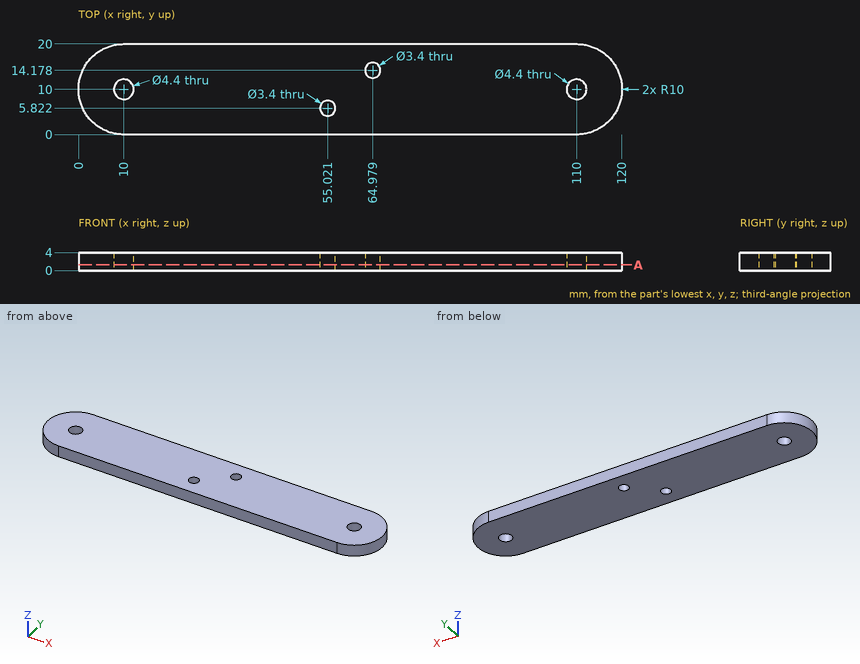
The figure shows three views and two pictorial views of one solid part (mm, origin at its lowest corner). Answer the questions. Give positions to 0.01 mm unless a question says otherwise; leave off trailing zeros. Order: outer loops, then holes, each group sorted by start corner. A loop starts at its lowest first (then second) coordinate and runs counter-clockwise, first axis right, second up. Notation, with made-up numbers: M -16.5,86 L 15.5,86 A21 cw 15.5,114 Z; hole C 58,-37 d3. An arc over 180 degrees is marked long. Return JSON: item names as keys, results as strings.
Q1. Each of these flat-tipped pins is pushed along its axis until it touches: pin 1 (4 mm diameter, centred on x = 10, y = 10, fed in from +Z); pin 2 (1.5 mm diameter, centred on y = 2, z = 2.5, fed in from -X). Where does it stop, or does it pass through?
Answer below:
{"pin 1": "passes through", "pin 2": "stops at x = 3.11"}
Q2. Find section A-A, the plane z = 1.3. Write down the section's boundary in (x, y), and give its area (3 significant figures).
Answer below:
{"outline": "M 10,0 L 110,0 A10 ccw 110,20 L 10,20 A10 ccw Z; hole C 10,10 d4.4; hole C 55.02,5.82 d3.4; hole C 64.98,14.18 d3.4; hole C 110,10 d4.4", "area": "2,270 mm^2"}
Q3. Find the intervals of material crossed by line 1 along Y through (x, z) = (110, 2.95); line 2 along Y through (x, z) = (108.5, 2.4); line 3 along Y through (x, z) = (115, 0.85), in increasing order. Write a range as [from, to].
Answer below:
{"line 1": "y = [0, 7.8], [12.2, 20]", "line 2": "y = [0, 8.39], [11.61, 20]", "line 3": "y = [1.34, 18.66]"}
